The listing builds one solid part. Answer for the finished solid, in the listing's coordinates (mm). Round coordinates to 2 decimals unless told otherwise and drop trailing zeros. Loops run counter-clockwise (first coordinate to the right, second up) from the corner with the lowest first, then second, coordinate; pieces in that order, holes last. Notation, with made-up numbers: (30, -20.75) -> (76, -20.75) arc R16 ccw to (76, -15.75) -> close; hole circle Ø3 at (38, -12.5). An arc over 180 degrees is marked (long way). Use a Markdown table: item, result. Add a question column.
Q1. Section B-B on z = -10 is taken. Give the vertices of the cut face in (x, y).
Q2. Section D-D on y = 0.35 is taken. Give the number of separate pieces and of enclosed holes in the cut face, then the cut area to 3 significant figures.
Q3. Consider line 1 (Z direction, x = -3, y = 0.9); line 2 (Z direction, x = 6.5, y = 0.55); line 3 (Z direction, x = 13, y = 0.8). Determine where each line is inside the solid, lowest interval first.
Q4. Section C-C on x = 11 is taken. Give the vertices of the cut face in (y, z), then the cut area to 3 significant figures.
Q5. For a pull along X with two mould halves and no side action, classify faces 1 (the cylindrical face through (0.1, 0.5, -30)), 2 (the flat face through (-9, 1, -9)), 3 (the cylindrical face through (-0.434, 0.493, 24.548)) as released by +X, released by -X, zero draft, split by the parting line, or undercut.
Q6. Section A-A on z = 0 is taken. Give the vertices of the cut face in (x, y), then the cut area to 3 significant figures.
from build123d import *

# Parameters (mm, degrees)
SKETCH1_R           = 23
BOSS_EXTRUDE1_DEPTH = 3
SKETCH2_R           = 12
CUT_EXTRUDE1_DEPTH  = 10
SKETCH3_R           = 1.75
BOSS_EXTRUDE2_DEPTH = 3
SKETCH4_R           = 2.8
CUT_EXTRUDE2_DEPTH  = 1
FILLET1_R           = 10
SKETCH5_R           = 31.123463038
CUT_EXTRUDE3_DEPTH  = 1
CUT_EXTRUDE4_DEPTH  = 1
SKETCH7_R           = 2.8
SKETCH7_R_2         = 2
BOSS_EXTRUDE3_DEPTH = 1


with BuildPart() as part:
    # Sketch1 → Boss-Extrude1 (new body)
    with BuildSketch(Plane(origin=(0, 0, 0), x_dir=(1, 0, 0), z_dir=(0, 1, 0))):
        Circle(SKETCH1_R)
    extrude(amount=BOSS_EXTRUDE1_DEPTH)

    # Sketch2 → Cut-Extrude1 (cut)
    with BuildSketch(Plane.XZ):
        Circle(SKETCH2_R)
    extrude(amount=-CUT_EXTRUDE1_DEPTH, mode=Mode.SUBTRACT)

    # Sketch3 → Boss-Extrude2 (add)
    with BuildSketch(Plane.XZ):
        with BuildLine():
            Line((-26.5, 3.5), (-22.732135843, 3.5))
            ThreePointArc((-22.732135843, 3.5), (-23, 0), (-22.732135843, -3.5))
            Line((-22.732135843, -3.5), (-26.5, -3.5))
            ThreePointArc((-26.5, -3.5), (-30, 0), (-26.5, 3.5))
        make_face()
        with Locations((-26.5, 0)):
            Circle(SKETCH3_R, mode=Mode.SUBTRACT)
        with BuildLine():
            Line((3.5, 26.5), (3.5, 22.732135843))
            ThreePointArc((3.5, 22.732135843), (0, 23), (-3.5, 22.732135843))
            Line((-3.5, 22.732135843), (-3.5, 26.5))
            ThreePointArc((-3.5, 26.5), (0, 30), (3.5, 26.5))
        make_face()
        with Locations((0, 26.5)):
            Circle(SKETCH3_R, mode=Mode.SUBTRACT)
        with BuildLine():
            Line((26.5, -3.5), (22.732135843, -3.5))
            ThreePointArc((22.732135843, -3.5), (23, 0), (22.732135843, 3.5))
            Line((22.732135843, 3.5), (26.5, 3.5))
            ThreePointArc((26.5, 3.5), (30, 0), (26.5, -3.5))
        make_face()
        with Locations((26.5, 0)):
            Circle(SKETCH3_R, mode=Mode.SUBTRACT)
        with BuildLine():
            Line((-3.5, -26.5), (-3.5, -22.732135843))
            ThreePointArc((-3.5, -22.732135843), (0, -23), (3.5, -22.732135843))
            Line((3.5, -22.732135843), (3.5, -26.5))
            ThreePointArc((3.5, -26.5), (0, -30), (-3.5, -26.5))
        make_face()
        with Locations((0, -26.5)):
            Circle(SKETCH3_R, mode=Mode.SUBTRACT)
    extrude(amount=-BOSS_EXTRUDE2_DEPTH)

    # Sketch4 → Cut-Extrude2 (cut)
    with BuildSketch(Plane.XZ):
        with Locations((-26.5, 0)):
            Circle(SKETCH4_R)
        with Locations((0, 26.5)):
            Circle(SKETCH4_R)
        with Locations((26.5, 0)):
            Circle(SKETCH4_R)
        with Locations((0, -26.5)):
            Circle(SKETCH4_R)
    extrude(amount=-CUT_EXTRUDE2_DEPTH, mode=Mode.SUBTRACT)

    # Fillet1
    fillet1_edges = [part.edges().sort_by_distance(p)[0] for p in [
        (3.5, 1.5, 22.732135843),
        (22.732135843, 1.5, 3.5),
        (22.732135843, 1.5, -3.5),
        (3.5, 1.5, -22.732135843),
        (-3.5, 1.5, -22.732135843),
        (-22.732135843, 1.5, -3.5),
        (-22.732135843, 1.5, 3.5),
        (-3.5, 1.5, 22.732135843),
    ]]
    fillet(fillet1_edges, radius=FILLET1_R)

    # Sketch5 → Cut-Extrude3 (cut)
    with BuildSketch(Plane(origin=(0, 3, 0), x_dir=(1, 0, 0), z_dir=(0, 1, 0))):
        Circle(SKETCH5_R)
    extrude(amount=-CUT_EXTRUDE3_DEPTH, mode=Mode.SUBTRACT)

    # Sketch6 → Cut-Extrude4 (cut)
    with BuildSketch(Plane(origin=(0, 2, 0), x_dir=(1, 0, 0), z_dir=(0, 1, 0))):
        with BuildLine():
            ThreePointArc((3.353997774, 27.500349406), (5.477838975, 23.697921815), (9.016591418, 21.15894797))
            ThreePointArc((9.016591418, 21.15894797), (16.263455967, 16.263455967), (21.15894797, 9.016591418))
            ThreePointArc((21.15894797, 9.016591418), (23.697921815, 5.477838975), (27.500349406, 3.353997774))
            ThreePointArc((27.500349406, 3.353997774), (30, 0), (27.500349406, -3.353997774))
            ThreePointArc((27.500349406, -3.353997774), (23.697921815, -5.477838975), (21.15894797, -9.016591418))
            ThreePointArc((21.15894797, -9.016591418), (16.263455967, -16.263455967), (9.016591418, -21.15894797))
            ThreePointArc((9.016591418, -21.15894797), (5.477838975, -23.697921815), (3.353997774, -27.500349406))
            ThreePointArc((3.353997774, -27.500349406), (0, -30), (-3.353997774, -27.500349406))
            ThreePointArc((-3.353997774, -27.500349406), (-5.477838975, -23.697921815), (-9.016591418, -21.15894797))
            ThreePointArc((-9.016591418, -21.15894797), (-16.263455967, -16.263455967), (-21.15894797, -9.016591418))
            ThreePointArc((-21.15894797, -9.016591418), (-23.697921815, -5.477838975), (-27.500349406, -3.353997774))
            ThreePointArc((-27.500349406, -3.353997774), (-30, 0), (-27.500349406, 3.353997774))
            ThreePointArc((-27.500349406, 3.353997774), (-23.697921815, 5.477838975), (-21.15894797, 9.016591418))
            ThreePointArc((-21.15894797, 9.016591418), (-16.263455967, 16.263455967), (-9.016591418, 21.15894797))
            ThreePointArc((-9.016591418, 21.15894797), (-5.477838975, 23.697921815), (-3.353997774, 27.500349406))
            ThreePointArc((-3.353997774, 27.500349406), (0, 30), (3.353997774, 27.500349406))
        make_face()
    extrude(amount=-CUT_EXTRUDE4_DEPTH, mode=Mode.SUBTRACT)

    # Sketch7 → Boss-Extrude3 (add)
    with BuildSketch(Plane.XZ):
        with Locations((0, 26.5)):
            Circle(SKETCH7_R)
        with Locations((0, 26.5)):
            Circle(SKETCH7_R_2, mode=Mode.SUBTRACT)
        with Locations((26.5, 0)):
            Circle(SKETCH7_R)
        with Locations((26.5, 0)):
            Circle(SKETCH7_R_2, mode=Mode.SUBTRACT)
        with Locations((0, -26.5)):
            Circle(SKETCH7_R)
        with Locations((0, -26.5)):
            Circle(SKETCH7_R_2, mode=Mode.SUBTRACT)
        with Locations((-26.5, 0)):
            Circle(SKETCH7_R)
        with Locations((-26.5, 0)):
            Circle(SKETCH7_R_2, mode=Mode.SUBTRACT)
    extrude(amount=-BOSS_EXTRUDE3_DEPTH)


solid = part.part
Checked values:
| question | item | result |
|---|---|---|
| 1 | outline | (-20.71, 0) -> (-6.63, 0) -> (-6.63, 1) -> (-20.71, 1) -> close; (6.63, 0) -> (20.71, 0) -> (20.71, 1) -> (6.63, 1) -> close |
| 2 | separate pieces | 1 |
| 2 | enclosed holes | 5 |
| 2 | area | 1,390 mm2 |
| 3 | line 1 | z = -28.3 to -11.62, 11.62 to 28.3 |
| 3 | line 2 | z = -22.71 to -10.09, 10.09 to 22.71 |
| 3 | line 3 | z = -18.97 to 18.97 |
| 4 | outline | (0, -20.2) -> (1, -20.2) -> (1, -4.8) -> (0, -4.8) -> close; (0, 4.8) -> (1, 4.8) -> (1, 20.2) -> (0, 20.2) -> close |
| 4 | area | 30.8 mm2 |
| 5 | face 1 | split by the parting line |
| 5 | face 2 | zero draft |
| 5 | face 3 | undercut |
| 6 | outline | (-30, 0) -> (-28.5, 0) -> (-28.5, 1) -> (-30, 1) -> close; (-24.5, 0) -> (-12, 0) -> (-12, 1) -> (-24.5, 1) -> close; (12, 0) -> (24.5, 0) -> (24.5, 1) -> (12, 1) -> close; (28.5, 0) -> (30, 0) -> (30, 1) -> (28.5, 1) -> close |
| 6 | area | 28.0 mm2 |
